CAD build for the part. Positions are in the model's coordinates, mm. A direction names the side the tool comes from. Give positions to 0.01 mm unless a question says otherwise; leave off trailing zeros. Order: outer loops, then holes, each group sorted by start corner. A loop starts at its lowest first (then second) coordinate and runs counter-clockwise, first axis right, second up.
Item 1: Band-saw the part on B-B on z = 41. Give the cut face in (x, y), plus the area to 3 significant figures.
Item 2: Flat gauge pins, fed straight in: P1, Ø2, axis at x = -117, y = 10, coming from the -Z side; P2, Ø2, axis at x = -22, z = -47.5, coming from the +Y side; P3, Ø4.5, axis at x = -115, z = -122.5, coming from the -Y side. Where does each tip first touch, or does it go through?
Item 3: Band-saw the part on D-D on z = 94. Give the cut face in (x, y), plus the area to 3 significant figures.
Item 4: Two-plate mould, pull along X, no slides. Class faces 5 (the flat face through (-120, -10.2, 103)), 6 (the flat face through (-150, 6, -2)), 7 (the flat face through (-134, 3.8, 12)): released by +X, released by -X, zero draft, split by the parting line, or undercut.
Item 5: Which spindle directions (+Z, -Z, +X, -X, +Y, -Y) get a long thin tool onto all of the face, cutting with end or side? Do faces 1 (the flat face through (-137, 11, 13)), 2 (the flat face through (-125, 13, -112)), 3 (the flat face through (0, 5.8, 128)), 4 (the cylindrical face through (-19.524, -7.564, 4.336)). Say none if no direction does.
Item 6: Wall check: L1, parallel to X at y = 4, z = -122.5; L2, parallel to X at y = 1.5, z = 125; L3, parallel to X at y = 14.5, z = -16. Give the ranges that are in metal, low to high.
Item 7: Band-saw the part on A-A on x = 69. Give the cut face in (y, z).
Item 8: Band-saw the part on C-C on z = -77. Give the cut face in (x, y).
```python
from build123d import *

# Parameters (mm, degrees)
SKETCH_1_W                 = 260
SKETCH_1_H                 = 265
EXTRUDE_577_DEPTH          = 5.8
SKETCH_17_W                = 260
SKETCH_17_H                = 15
EXTRUDE_803_DEPTH          = 10
SKETCH_19_W                = 265
SKETCH_19_H                = 15.8
EXTRUDE_982_DEPTH          = 20
SKETCH_20_W                = 265
SKETCH_20_H                = 15.8
EXTRUDE_1186_DEPTH         = 20
SKETCH_22_W                = 75
SKETCH_22_H                = 15
CUT_EXTRUDE_1675_DEPTH     = 5.4
SKETCH_25_W                = 5
SKETCH_25_H                = 40.1
EXTRUDE_1_DEPTH            = 10
SKETCH_26_W                = 250
SKETCH_26_H                = 25.1
EXTRUDE_1_2_DEPTH          = 4.9
HOLE_WIZARD_M6_D           = 5
HOLE_WIZARD_M6_CSINK_D     = 6.05
HOLE_WIZARD_M6_CSINK_ANGLE = 90
SKETCH_27_W                = 210
SKETCH_27_H                = 25.1
EXTRUDE_3711_DEPTH         = 5.1
CUT_EXTRUDE_1_DEPTH        = 329.338072724
CUT_EXTRUDE_2_REACH        = 306.917
SKETCH_29_R                = 5.1
CUT_EXTRUDE_4572_DEPTH     = 5.1
HOLE_WIZARD_3_D            = 2.5
HOLE_WIZARD_3_CSINK_D      = 3.05
HOLE_WIZARD_3_CSINK_ANGLE  = 90
SKETCH_32_W                = 250
SKETCH_32_H                = 15
EXTRUDE_3_DEPTH            = 4.9
SKETCH_38_W                = 100
SKETCH_38_H                = 15
EXTRUDE_2_DEPTH            = 5.1
SKETCH_34_W                = 300
SKETCH_34_H                = 265
EXTRUDE_4_DEPTH            = 5
SKETCH_33_R                = 20
EXTRUDE_7147_DEPTH         = 5.2
SKETCH_36_W                = 7
SKETCH_36_H                = 32
SKETCH_36_W_2              = 26
SKETCH_36_H_2              = 7
CUT_EXTRUDE_7671_DEPTH     = 12
FILLET_2_R                 = 3
FILLET_3_R                 = 6
SKETCH_39_W                = 20
SKETCH_39_H                = 20
CUT_EXTRUDE_1_2_DEPTH      = 2.5
FILLET_4_R                 = 1.5


with BuildPart() as part:
    # Эскиз1 → Extrude 577 (new body)
    with BuildSketch(Plane(origin=(0, 0, 0), x_dir=(1, 0, 0), z_dir=(0, 1, 0))):
        Rectangle(SKETCH_1_W, SKETCH_1_H)
    extrude(amount=EXTRUDE_577_DEPTH)

    # Эскиз17 → Extrude 803 (add)
    with BuildSketch(Plane(origin=(0, 5.8, 0), x_dir=(1, 0, 0), z_dir=(0, 1, 0))):
        with Locations((0, -125)):
            Rectangle(SKETCH_17_W, SKETCH_17_H)
    extrude(amount=EXTRUDE_803_DEPTH)

    # Эскиз19 → Extrude 982 (add)
    with BuildSketch(Plane(origin=(130, 0, 0), x_dir=(0, 0, -1), z_dir=(1, 0, 0))):
        with Locations((0, 7.9)):
            Rectangle(SKETCH_19_W, SKETCH_19_H)
    extrude(amount=EXTRUDE_982_DEPTH)

    # Эскиз20 → Extrude 1186 (add)
    with BuildSketch(Plane.ZY.offset(130)):
        with Locations((0, 7.9)):
            Rectangle(SKETCH_20_W, SKETCH_20_H)
    extrude(amount=EXTRUDE_1186_DEPTH)

    # Эскиз22 → Cut-Extrude 1675 (cut)
    with BuildSketch(Plane(origin=(0, 15.8, 0), x_dir=(1, 0, 0), z_dir=(0, 1, 0))):
        with Locations((-87.5, -125)):
            Rectangle(SKETCH_22_W, SKETCH_22_H)
        with Locations((87.5, -125)):
            Rectangle(SKETCH_22_W, SKETCH_22_H)
    extrude(amount=-CUT_EXTRUDE_1675_DEPTH, mode=Mode.SUBTRACT)

    # Эскиз25 → Extrude 1 (add)
    with BuildSketch(Plane(origin=(0, 5.8, 0), x_dir=(1, 0, 0), z_dir=(0, 1, 0))):
        with Locations((127.5, 112.45)):
            Rectangle(SKETCH_25_W, SKETCH_25_H)
        with Locations((-127.5, 112.45)):
            Rectangle(SKETCH_25_W, SKETCH_25_H)
    extrude(amount=EXTRUDE_1_DEPTH)

    # Эскиз26 → Extrude 1 2 (add)
    with BuildSketch(Plane(origin=(0, 5.8, 0), x_dir=(1, 0, 0), z_dir=(0, 1, 0))):
        with Locations((0, 119.95)):
            Rectangle(SKETCH_26_W, SKETCH_26_H)
    extrude(amount=EXTRUDE_1_2_DEPTH)

    # Крепление для уровня M6 (through all)
    with Locations(Plane(origin=(0, 10.7, 0), x_dir=(1, 0, 0), z_dir=(0, 1, 0))):
        with Locations((-115, 122.5), (115, 122.5)):
            CounterSinkHole(HOLE_WIZARD_M6_D / 2, HOLE_WIZARD_M6_CSINK_D / 2, counter_sink_angle=HOLE_WIZARD_M6_CSINK_ANGLE)

    # Эскиз27 → Extrude 3711 (add)
    with BuildSketch(Plane(origin=(0, 10.7, 0), x_dir=(1, 0, 0), z_dir=(0, 1, 0))):
        with Locations((0, 119.95)):
            Rectangle(SKETCH_27_W, SKETCH_27_H)
    extrude(amount=EXTRUDE_3711_DEPTH)

    # Эскиз28 → Cut-Extrude 1 (cut, through all)
    with BuildSketch(Plane(origin=(150, 0, 0), x_dir=(0, 0, -1), z_dir=(1, 0, 0))):
        with BuildLine():
            Line((-20.05, 10.8), (-5.05, 10.8))
            ThreePointArc((-5.05, 10.8), (-2.55, 8.3), (-5.05, 5.8))
            Line((-5.05, 5.8), (-20.05, 5.8))
            ThreePointArc((-20.05, 5.8), (-22.55, 8.3), (-20.05, 10.8))
        make_face()
    extrude(amount=-CUT_EXTRUDE_1_DEPTH, mode=Mode.SUBTRACT)

    # Эскиз37 → Регулировка-2 (cut, up to next)
    with BuildSketch(Plane.XY.offset(132.5), mode=Mode.PRIVATE) as cut_extrude_2_sk1:
        with BuildLine():
            Line((-5, 10.8), (5, 10.8))
            ThreePointArc((5, 10.8), (7.5, 8.3), (5, 5.8))
            Line((5, 5.8), (-5, 5.8))
            ThreePointArc((-5, 5.8), (-7.5, 8.3), (-5, 10.8))
        make_face()
    cut_extrude_2_tool1 = extrude(cut_extrude_2_sk1.sketch, amount=-CUT_EXTRUDE_2_REACH, mode=Mode.PRIVATE) & part.part
    add(cut_extrude_2_tool1.solids().sort_by_distance((0, 8.3, 132.5))[0], mode=Mode.SUBTRACT)

    # Эскиз29 → Cut-Extrude 4572 (cut)
    with BuildSketch(Plane(origin=(0, 10.4, 0), x_dir=(1, 0, 0), z_dir=(0, 1, 0))):
        with Locations(Location((-105, -125, 0), (0, 0, 270))):
            Circle(SKETCH_29_R)
        with Locations(Location((105, -125, 0), (0, 0, 270))):
            Circle(SKETCH_29_R)
    extrude(amount=-CUT_EXTRUDE_4572_DEPTH, mode=Mode.SUBTRACT)

    # КреплениеМагнитов-М3 (through all)
    with Locations(Plane(origin=(0, 5.3, 0), x_dir=(1, 0, 0), z_dir=(0, 1, 0))):
        with Locations((-105, -125), (105, -125)):
            CounterSinkHole(HOLE_WIZARD_3_D / 2, HOLE_WIZARD_3_CSINK_D / 2, counter_sink_angle=HOLE_WIZARD_3_CSINK_ANGLE)

    # Эскиз32 → Бобышка-Вытянуть3 (add)
    with BuildSketch(Plane(origin=(0, 5.8, 0), x_dir=(1, 0, 0), z_dir=(0, 1, 0))):
        with Locations((0, 99.9)):
            Rectangle(SKETCH_32_W, SKETCH_32_H)
    extrude(amount=EXTRUDE_3_DEPTH)

    # Эскиз38 → НаправляющийВынос-2 (add)
    with BuildSketch(Plane(origin=(0, 10.7, 0), x_dir=(1, 0, 0), z_dir=(0, 1, 0))):
        with Locations((0, 99.9)):
            Rectangle(SKETCH_38_W, SKETCH_38_H)
    extrude(amount=EXTRUDE_2_DEPTH)

    # Эскиз34 → Бобышка-Вытянуть4 (add)
    with BuildSketch(Plane.XZ):
        Rectangle(SKETCH_34_W, SKETCH_34_H)
    extrude(amount=EXTRUDE_4_DEPTH)

    # Эскиз33 → Extrude 7147 (add)
    with BuildSketch(Plane.XZ.offset(5)):
        with Locations(Location((0, 0, 0), (0, 0, 270))):
            Circle(SKETCH_33_R)
        with Locations(Location((-120, 102.5, 0), (0, 0, 270))):
            Circle(SKETCH_33_R)
        with Locations(Location((120, 102.5, 0), (0, 0, 270))):
            Circle(SKETCH_33_R)
        with Locations(Location((120, -92.5, 0), (0, 0, 270))):
            Circle(SKETCH_33_R)
        with Locations(Location((-120, -92.5, 0), (0, 0, 270))):
            Circle(SKETCH_33_R)
    extrude(amount=EXTRUDE_7147_DEPTH)

    # Эскиз36 → Cut-Extrude 7671 (cut)
    with BuildSketch(Plane(origin=(0, 15.8, 0), x_dir=(1, 0, 0), z_dir=(0, 1, 0))):
        with Locations((133.5, -12.55)):
            Rectangle(SKETCH_36_W, SKETCH_36_H)
        with Locations((-133.5, -12.55)):
            Rectangle(SKETCH_36_W, SKETCH_36_H)
        with Locations((0, -121)):
            Rectangle(SKETCH_36_W_2, SKETCH_36_H_2)
    extrude(amount=-CUT_EXTRUDE_7671_DEPTH, mode=Mode.SUBTRACT)

    # Скругление2
    fillet_2_edges = [part.edges().sort_by_distance(p)[0] for p in [
        (50, 13.25, -107.4),
        (-50, 13.25, -107.4),
        (137, 9.8, -3.45),
        (137, 9.8, 28.55),
        (130, 4.8, 28.55),
        (130, 4.8, -3.45),
        (-130, 4.8, -3.45),
        (-130, 4.8, 28.55),
        (-137, 9.8, 28.55),
        (-137, 9.8, -3.45),
        (-13, 9.8, 124.5),
        (-13, 4.8, 117.5),
        (13, 4.8, 117.5),
        (13, 9.8, 124.5),
    ]]
    fillet(fillet_2_edges, radius=FILLET_2_R)

    # Скругление3
    fillet_3_edges = [part.edges().sort_by_distance(p)[0] for p in [
        (130, 10.8, 117.5),
        (130, 10.8, -92.4),
        (-130, 10.8, 117.5),
        (-130, 10.8, -92.4),
    ]]
    fillet(fillet_3_edges, radius=FILLET_3_R)

    # Эскиз39 → Cut-Extrude 1 2 (cut)
    with BuildSketch(Plane(origin=(0, 10.7, 0), x_dir=(1, 0, 0), z_dir=(0, 1, 0))):
        with Locations((-115, 122.5)):
            Rectangle(SKETCH_39_W, SKETCH_39_H)
        with Locations((115, 122.5)):
            Rectangle(SKETCH_39_W, SKETCH_39_H)
    extrude(amount=-CUT_EXTRUDE_1_2_DEPTH, mode=Mode.SUBTRACT)

    # Скругление4
    fillet_4_edges = [part.edges().sort_by_distance(p)[0] for p in [
        (-105, 9.45, -112.5),
        (-125, 9.45, -112.5),
        (105, 9.45, -112.5),
        (125, 9.45, -112.5),
    ]]
    fillet(fillet_4_edges, radius=FILLET_4_R)


solid = part.part
```
The answers:
1. outline: (-150, -5) - (150, -5) - (150, 15.8) - (130, 15.8) - (130, 5.8) - (-130, 5.8) - (-130, 15.8) - (-150, 15.8) - close
1. area: 3,640 mm2
2. P1: stops at z = -112.5
2. P2: stops at y = 5.8
2. P3: stops at y = -5
3. outline: (-150, -5) - (-138.1, -5) - (-138.1, -10.2) - (-101.9, -10.2) - (-101.9, -5) - (101.9, -5) - (101.9, -10.2) - (138.1, -10.2) - (138.1, -5) - (150, -5) - (150, 15.8) - (130, 15.8) - (130, 5.8) - (-130, 5.8) - (-130, 15.8) - (-150, 15.8) - close
3. area: 4,020 mm2
4. face 5: zero draft
4. face 6: released by -X
4. face 7: undercut
5. face 1: +Y
5. face 2: -Z, +Y
5. face 3: +Z
5. face 4: -Y
6. L1: x = -150 to -117.5, -112.5 to 112.5, 117.5 to 150
6. L2: x = -150 to -106.25, -103.75 to 103.75, 106.25 to 150
6. L3: x = -150 to -130, 130 to 150
7. outline: (-5, -132.5) - (15.8, -132.5) - (15.8, -107.4) - (10.7, -107.4) - (10.7, -92.4) - (5.8, -92.4) - (5.8, 117.5) - (10.4, 117.5) - (10.4, 132.5) - (-5, 132.5) - close
8. outline: (-150, -5) - (-132.64, -5) - (-132.64, -10.2) - (-107.36, -10.2) - (-107.36, -5) - (107.36, -5) - (107.36, -10.2) - (132.64, -10.2) - (132.64, -5) - (150, -5) - (150, 15.8) - (130, 15.8) - (130, 5.8) - (-130, 5.8) - (-130, 15.8) - (-150, 15.8) - close
